```python
from build123d import *

# Parameters (mm, degrees)
SKETCH1_W           = 42
SKETCH1_H           = 42
BOSS_EXTRUDE1_DEPTH = 5
FILLET1_R           = 5
SKETCH2_R           = 15
BOSS_EXTRUDE2_DEPTH = 2.5
SKETCH3_R           = 3
BOSS_EXTRUDE3_DEPTH = 22.5
BOSS_EXTRUDE5_DEPTH = 64
CHAMFER1_SIZE       = 0.5


with BuildPart() as part:
    # Sketch1 → Boss-Extrude1 (new body)
    with BuildSketch(Plane.XY):
        Rectangle(SKETCH1_W, SKETCH1_H)
    extrude(amount=BOSS_EXTRUDE1_DEPTH)

    # Fillet1
    fillet1_edges = [part.edges().sort_by_distance(p)[0] for p in [
        (21, -21, 2.5),
        (-21, -21, 2.5),
        (-21, 21, 2.5),
        (21, 21, 2.5),
    ]]
    fillet(fillet1_edges, radius=FILLET1_R)

    # Sketch2 → Boss-Extrude2 (add)
    with BuildSketch(Plane.XY.offset(5)):
        Circle(SKETCH2_R)
    extrude(amount=BOSS_EXTRUDE2_DEPTH)

    # Sketch3 → Boss-Extrude3 (add)
    with BuildSketch(Plane.XY.offset(7.5)):
        with Locations(Location((0, 0, 0), (0, 0, 180))):
            Circle(SKETCH3_R)
    extrude(amount=BOSS_EXTRUDE3_DEPTH)

    # Sketch4 → Boss-Extrude5 (add)
    with BuildSketch(Plane(origin=(0, 0, 0), x_dir=(-1, 0, 0), z_dir=(0, 0, -1))):
        with BuildLine():
            Line((-21, -16), (-21, 16))
            ThreePointArc((-21, 16), (-19.535533906, 19.535533906), (-16, 21))
            Line((-16, 21), (16, 21))
            ThreePointArc((16, 21), (19.535533906, 19.535533906), (21, 16))
            Line((21, 16), (21, -16))
            ThreePointArc((21, -16), (19.535533906, -19.535533906), (16, -21))
            Line((16, -21), (-16, -21))
            ThreePointArc((-16, -21), (-19.535533906, -19.535533906), (-21, -16))
        make_face()
    extrude(amount=BOSS_EXTRUDE5_DEPTH)

    # Chamfer1
    chamfer1_edges = [part.edges().sort_by_distance(p)[0] for p in [
        (3, 0, 30),
    ]]
    chamfer(chamfer1_edges, length=CHAMFER1_SIZE)


solid = part.part
```
The listing builds one solid part. Answer for the finished solid, in the listing's coordinates (mm). A direction names the side the tool comes from. Coordinates: 2 decimals unless noted, no trailing zeros. Loops run counter-clockwise (first coordinate to the right, second up) from the corner with the lowest first, then second, coordinate; pieces in that order, holes last. Notation, with made-up numbers: (82.25, 44.5) - (128.25, 44.5) arc R19 cw to (128.25, 75.5) - close; hole circle Ø7 at (63, 79). An arc over 180 degrees is marked (long way). Use a Markdown table: item, result. Add a question column.
1) For faces 4 (the cylindrical face through (-14.985, 0.66, 6.232)), 5 (the flat face through (0, 21, -29)), determine the directions among +Z, -Z, +X, -X, +Y, -Y from which every point of the face is accessible in a straight line to the end or side of a thin tool.
2) The mould has two halves that part along Z. Classify faces 1 (the flat face through (-10, 14, 5)), 2 (the flat face through (0, 0, -64)), 3 (the flat face through (0, -21, -29)): released by +Z, released by -Z, zero draft, split by the parting line, or undercut.
3) The part is cut by section C-C, the plane x = 7. Give the vertices of the cut face in (y, z), and give its area (3 significant figures).
4) The part is cut by section D-D, the plane y = -12.5. Give the vertices of the cut face in (x, z), and give its area (3 significant figures).
5) Given pin 1 (10 mm diameter, centred on x = -7.5, y = 6, fed in from +Z), flat-ended and moving along its own axis, determine where the tip first touches the part or whether it passes through.
6) The part is cut by section A-A, the plane x = 0. Give the vertices of the cut face in (y, z).
7) Find the intervals of material crossed by line 1 (Z direction, x = -5, y = 10); line 2 (Z direction, x = -12, y = 10); line 3 (Y direction, x = 0, z = 6), in increasing order.
Here are the results:
| question | item | result |
|---|---|---|
| 1 | face 4 | +Z |
| 1 | face 5 | +Z, -Z, +X, -X, +Y |
| 2 | face 1 | released by +Z |
| 2 | face 2 | released by -Z |
| 2 | face 3 | zero draft |
| 3 | outline | (-21, -64) - (21, -64) - (21, 5) - (13.27, 5) - (13.27, 7.5) - (-13.27, 7.5) - (-13.27, 5) - (-21, 5) - close |
| 3 | area | 2,960 mm^2 |
| 4 | outline | (-21, -64) - (21, -64) - (21, 5) - (8.29, 5) - (8.29, 7.5) - (-8.29, 7.5) - (-8.29, 5) - (-21, 5) - close |
| 4 | area | 2,940 mm^2 |
| 5 | pin 1 | stops at z = 7.5 |
| 6 | outline | (-21, -64) - (21, -64) - (21, 5) - (15, 5) - (15, 7.5) - (3, 7.5) - (3, 29.5) - (2.5, 30) - (-2.5, 30) - (-3, 29.5) - (-3, 7.5) - (-15, 7.5) - (-15, 5) - (-21, 5) - close |
| 7 | line 1 | z = -64 to 7.5 |
| 7 | line 2 | z = -64 to 5 |
| 7 | line 3 | y = -15 to 15 |
